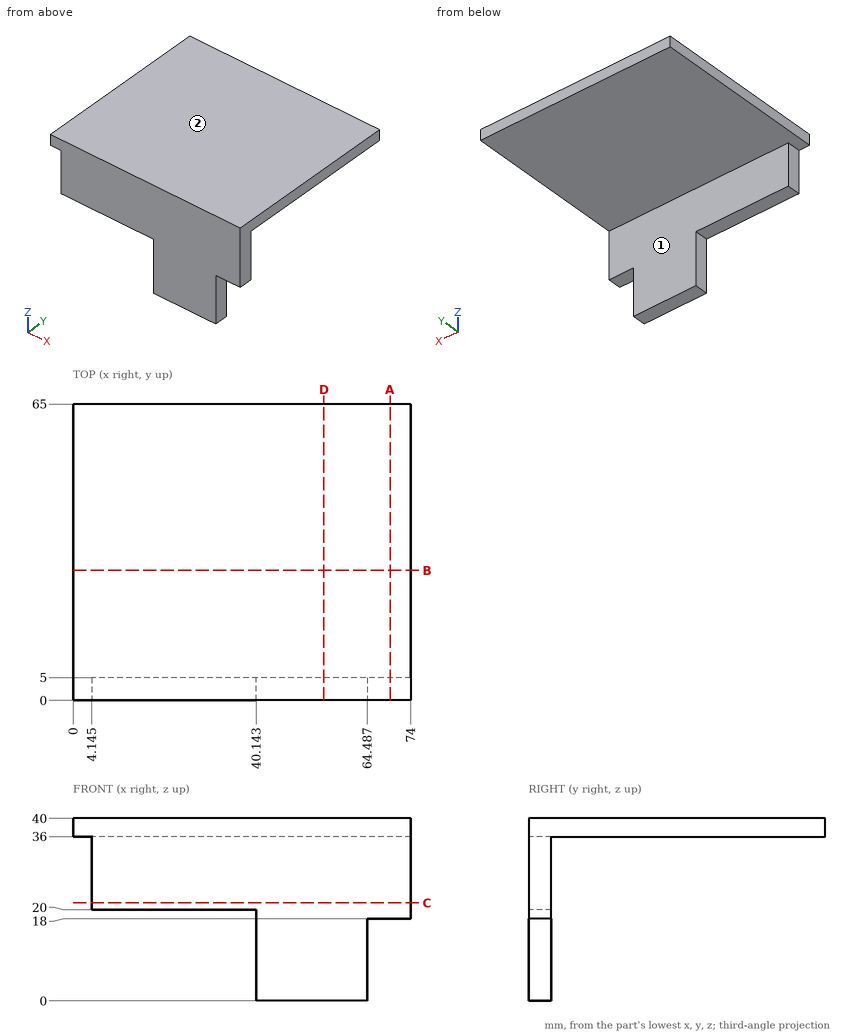
Geometry check sheet. Reference: drawing and pictorial views, mm from the part's lowest x, y, z. A direction names the side the tool comes from. Round coordinates to 2 decimals unless told otherwise and drop trailing zeros. Loops run counter-clockwise (first coordinate to the right, second up) from the corner with the lowest first, then second, coordinate; pieces in that order, holes last.
1. Sectioned sample at B-B on y = 28.5. Record the boundary of the cut face in (x, z).
2. Set-up check for the marked faces 1 and 2: record each of +Z, -Z, +X, -X, +Y, -Y from which the full face is reachable in a straight line by a thin tool's end or side.
3. Sectioned sample at D-D on x = 55. Record the boundary of the cut face in (y, z), and give its area (3 significant figures).
4. Gauge pin test, flat ends, axial feed: pin 1 Ø5 at (x, z) = (61, 17.5) entering from +Y; pin 2 Ø4 at (x, z) = (50, 13) entering from -Y; pin 3 Ø2.5 at (y, z) = (3.5, 31.5) entering from -X (1 decimal); pin 4 Ø19.5 at (x, y) = (41, 30) entering from -Z. Record the tip position at first contact, or that the pin passes through.
5. Scan lines: probe 1 along Z at (x, y) = (27.5, 43); probe 2 along Y at (x, z) = (45, 18). Record each from-to range of solid material in increasing order.
6. Sectioned sample at C-C on z = 21.5. Record the boundary of the cut face in (x, y) (1 decimal), and give its area (3 significant figures).
7. Sectioned sample at A-A on x = 69.5. Record the boundary of the cut face in (y, z).
Recorded:
1. outline: (0, 36) - (74, 36) - (74, 40) - (0, 40) - close
2. face 1: -Z, +X, -X, +Y
2. face 2: +Z, +X, -X, +Y, -Y
3. outline: (0, 0) - (5, 0) - (5, 36) - (65, 36) - (65, 40) - (0, 40) - close
3. area: 440 mm2
4. pin 1: stops at y = 5
4. pin 2: stops at y = 0
4. pin 3: stops at x = 4.1
4. pin 4: stops at z = 36
5. probe 1: z = 36 to 40
5. probe 2: y = 0 to 5
6. outline: (4.1, 0) - (74, 0) - (74, 5) - (4.1, 5) - close
6. area: 349 mm2
7. outline: (0, 18) - (5, 18) - (5, 36) - (65, 36) - (65, 40) - (0, 40) - close
